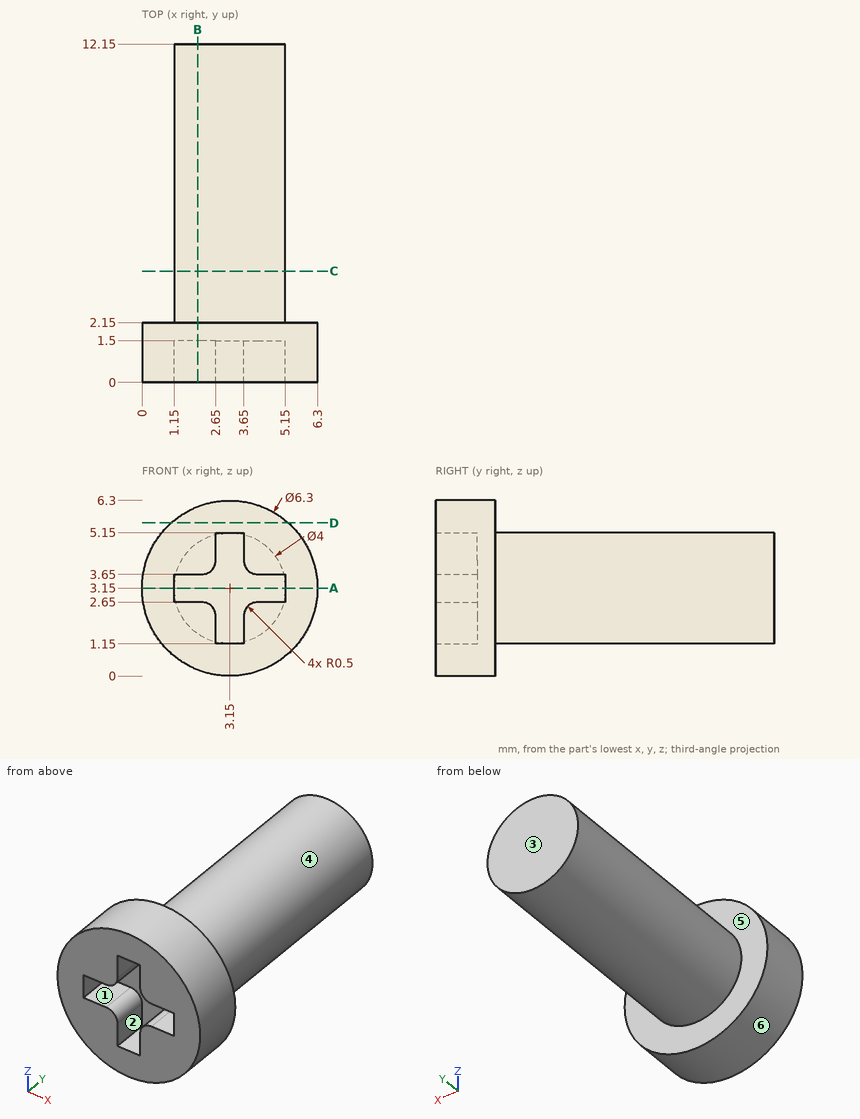
Drawing for the job (mm, zero at the part's lowest x, y, z). A direction names the side the tool comes from. Round coordinates to 2 decimals unless told otherwise and drop trailing zeros. Write each loop counter-clockwise with the first axis right and the second up, starting at its lowest first coordinate (ties: lowest second). Pieces come first, ordered by that corner, then holes. Notation, with made-up numbers: (-21, 75) - (-6, 75) arc R11 cw to (-6, 92) - close; hole circle Ø8 at (-21.75, 1). An arc over 180 degrees is marked (long way). Return JSON: item names as keys, results as strings. Group by question number.
Item 1: Flat gauge pins, fed straight in: pin 1 Ø1.1 at (y, z) = (1, 1.5) entering from +X; pin 2 Ø1.5 at (x, z) = (1, 5.5) entering from +Y; pin 3 Ø0.8 at (y, z) = (1, 4.5) entering from +X. Where does each tip first touch, or does it go through?
Item 2: 3-axis set-ups, long thin cutter, end or side, ignore diameter. For the marked faces 5 and 6: which of +Z, -Z, +X, -X, +Y, -Y reach the whole face in a straight line?
Item 3: Band-saw the part on D-D on z = 5.5. List the corners of the cut face in (x, y).
Item 4: Band-saw the part on A-A on z = 3.15. List the corners of the cut face in (x, y), plus the area to 3 significant figures.
Item 5: Mould opens along Z. For the marked faces 1, 2, 3 and 4 say: +Z half, -Z half, draft (parallel to the pull), parting line (faces both ways), or undercut.
Item 6: Band-saw the part on B-B on x = 2. List the corners of the cut face in (y, z).
Item 7: Probe probe 1 along Y at (x, z) = (4.75, 0.5); probe 2 along X at (y, z) = (3.75, 3.25); probe 3 along Y at (x, z) = (2.5, 2.75). List the from-to ranges inside material, lowest first.
Item 8: Band-saw the part on C-C on y = 4. List the corners of the cut face in (x, z), plus the area to 3 significant figures.
Resolved:
{
 "1": {"pin 1": "stops at x = 6.1", "pin 2": "stops at y = 2.15", "pin 3": "stops at x = 6.15"},
 "2": {"face 5": "+Y", "face 6": "+Y, -Y"},
 "3": {"outline": "(1.05, 0) - (5.25, 0) - (5.25, 2.15) - (1.05, 2.15) - close"},
 "4": {"outline": "(0, 0) - (1.15, 0) - (1.15, 1.5) - (5.15, 1.5) - (5.15, 0) - (6.3, 0) - (6.3, 2.15) - (5.15, 2.15) - (5.15, 12.15) - (1.15, 12.15) - (1.15, 2.15) - (0, 2.15) - close", "area": "47.5 mm²"},
 "5": {"face 1": "undercut", "face 2": "undercut", "face 3": "draft", "face 4": "parting line"},
 "6": {"outline": "(0, 0.22) - (2.15, 0.22) - (2.15, 1.51) - (12.15, 1.51) - (12.15, 4.79) - (2.15, 4.79) - (2.15, 6.08) - (0, 6.08) - (0, 3.65) - (1.5, 3.65) - (1.5, 2.65) - (0, 2.65) - close"},
 "7": {"probe 1": "y = 0 to 2.15", "probe 2": "x = 1.15 to 5.15", "probe 3": "y = 1.5 to 12.15"},
 "8": {"outline": "circle Ø4 at (3.15, 3.15)", "area": "12.6 mm²"}
}
